Build history of the part. All positions in model axes, mm. Face numbers are marked on the shaded views. A direction names the side the tool comes from. Give positions to 0.01 mm unless a question says otherwise; leave off trailing zeros. Loops run counter-clockwise (first coordinate to the right, second up) from the corner with the lowest first, then second, coordinate; pieces in that order, holes last. Notation, with made-up numbers: M 33,78.25 L 62,78.25 A9 cw 62,93.25 Z; hole C 32,-17 d1. An arc over 180 degrees is marked long. Put each result on its own line as item: value.
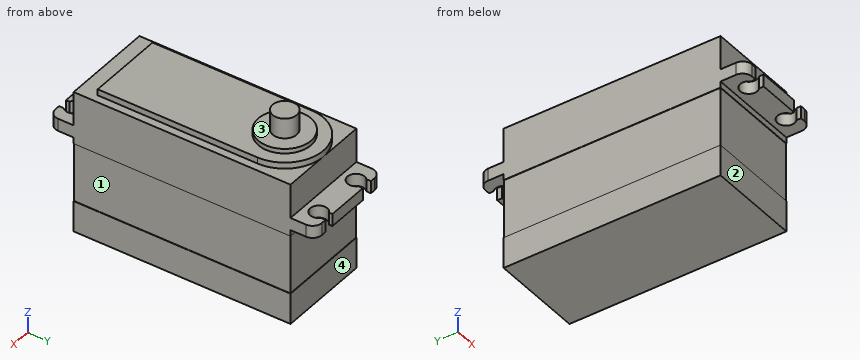
Autodesk Inventor part; units mm, degrees
ref_plane "Work Plane1" through (0, 0, 31) normal (0, 0, 1) x (1, 0, 0)
ref_plane "YZ Plane" through (0, 0, 0) normal (1, 0, 0) x (0, 1, 0)
ref_plane "XZ Plane" through (0, 0, 0) normal (0, 1, 0) x (-1, 0, 0)
sketch "Sketch1" plane through (0, 0, 0) normal (0, 0, 1) x (1, 0, 0)
  line L0 (0, 0) -> (-30, 0)
  line L1 (-30, 0) -> (-30, -70)
  line L2 (-30, -70) -> (0, -70)
  line L3 (0, -70) -> (0, 0)
  dimension "d0" = 30
  dimension "d1" = 70
extrude "Extrusion1" add sketch "Sketch1" along normal blind 10
sketch "Sketch2" plane through (0, 0, 10) normal (0, 0, 1) x (1, 0, 0)
  line L0 (-30, 0) -> (-30, -70)
  line L1 (-30, -70) -> (0, -70)
  line L2 (0, -70) -> (0, 0)
  line L3 (0, 0) -> (-30, 0)
  line L4 (0, 0) -> (-30, 0)
  line L5 (-30, -70) -> (0, -70)
  line L6 (-0.1, -70) -> (-0.1, -0.1)
  line L7 (-0.1, -0.1) -> (-30, -0.1)
  line L8 (-29.9, 0) -> (-29.9, -70)
  line L9 (-30, -69.9) -> (0, -69.9)
  point P0 (-29.9, -69.9)
  point P1 (-0.1, -69.9)
  point P2 (-29.9, -0.1)
  dimension "d29" = 0.1
  dimension "d30" = 0.1
  dimension "d31" = 0.1
extrude "Extrusion2" add sketch "Sketch2" along normal blind 19 contours L7 L6 L9 L8
sketch "Sketch3" plane through (0, 0, 29) normal (0, 0, 1) x (1, 0, 0)
  line L0 (-30, -70) -> (0, -70)
  line L1 (-30, 0) -> (-30, -70)
  line L2 (0, -70) -> (0, 0)
  line L3 (-30, -70) -> (0, -70)
  line L4 (0, 0) -> (-30, 0)
  line L5 (0, 0) -> (-30, 0)
  line L6 (0, -70) -> (0, 0)
  point P0 (-0.01, -70)
  point P1 (-0.01, 0)
extrude "Extrusion3" add sketch "Sketch3" along normal blind 19
sketch "Sketch4" plane through (0, 0, 48) normal (0, 0, 1) x (1, 0, 0)
  circle A0 centre (-15, -12.5) radius 8.5
  line L0 (0, 0) -> (-30, 0)
  dimension "d8" = 17
  dimension "d26" = 12.5
extrude "Extrusion4" add sketch "Sketch4" along normal blind 1.5
sketch "Sketch5" plane through (-15, -12.5, 49.5) normal (0, 0, 1) x (1, 0, 0)
  circle A0 centre (0, 0) radius 3.9
  point P0 (15, 12.5)
  dimension "d11" = 7.8
extrude "Extrusion5" add sketch "Sketch5" along normal blind 6.5
ref_plane "Work Plane1" through (0, 0, 31) normal (0, 0, 1) x (1, 0, 0)
sketch "Sketch6" plane through (0, 0, 31) normal (0, 0, 1) x (1, 0, 0)
  line L0 (-30, -70) -> (0, -70)
  line L1 (0, -70) -> (-30, -70)
  line L2 (-30, -70) -> (-30, -78)
  line L3 (0, -78) -> (0, -70)
  arc A0 (-4.6303, -76.5166) -> (-7.7916, -76.9278) centre (-6.5, -74.5) ccw
  arc A1 (-21.6303, -76.5166) -> (-25.3697, -76.5166) centre (-23.5, -74.5) ccw
  line L4 (-4.6303, -76.5166) -> (-4.6303, -78)
  line L5 (-7.7916, -76.9278) -> (-7.7916, -78)
  line L6 (-4.6303, -78) -> (0, -78)
  line L7 (-30, -78) -> (-25.3697, -78)
  line L8 (-21.6303, -78) -> (-7.7916, -78)
  line L9 (-21.6303, -76.5166) -> (-21.6303, -78)
  line L10 (-25.3697, -76.5166) -> (-25.3697, -78)
  line L11 (0, -70) -> (0, 0)
  line L12 (0, -35) -> (-30, -35) construction
  line L13 (-30, 0) -> (0, 0)
  line L14 (0, 0) -> (-30, 0)
  line L15 (-30, 0) -> (-30, 8)
  line L16 (0, 8) -> (0, 0)
  arc A2 (-7.7916, 6.9278) -> (-4.6303, 6.5166) centre (-6.5, 4.5) ccw
  arc A3 (-25.3697, 6.5166) -> (-21.6303, 6.5166) centre (-23.5, 4.5) ccw
  line L17 (-4.6303, 6.5166) -> (-4.6303, 8)
  line L18 (-7.7916, 6.9278) -> (-7.7916, 8)
  line L19 (-4.6303, 8) -> (0, 8)
  line L20 (-30, 8) -> (-25.3697, 8)
  line L21 (-21.6303, 8) -> (-7.7916, 8)
  line L22 (-21.6303, 6.5166) -> (-21.6303, 8)
  line L23 (-25.3697, 6.5166) -> (-25.3697, 8)
  point P0 (-0.01, -70)
  dimension "d15" = 30
  dimension "d16" = 8
  dimension "d17" = 5.5
  dimension "d18" = 5.5
  dimension "d21" = 6.5
  dimension "d22" = 6.5
extrude "Extrusion6" add sketch "Sketch6" along normal blind 4
fillet "Fillet1" radius 3 4 edges at (-30, 8, 33) (0, 8, 33) (-30, -78, 33) (0, -78, 33)
sketch "Sketch7" plane through (0, 0, 48) normal (0, 0, 1) x (1, 0, 0)
  point P0 (0, 0)
sketch "Sketch8" plane through (0, 0, 48) normal (0, 0, 1) x (1, 0, 0)
  circle A0 centre (-15, -12.5) radius 8.5
  circle A1 centre (-15, -12.5) radius 12.5
  line L0 (0, -70) -> (0, 0)
  line L1 (-2.5, -64) -> (-27.5, -64)
  line L2 (-30, 0) -> (-30, -70)
  line L3 (-2.5, -12.5) -> (-2.5, -64)
  line L4 (-27.5, -12.5) -> (-27.5, -64)
  line L5 (-30, -70) -> (0, -70)
  line L6 (0, 0) -> (-30, 0)
  point P0 (-15, 0)
extrude "Extrusion7" cut sketch "Sketch8" against normal blind 2 contours L6 L0 L5 L2
properties part number "serwo 30x70"
Q1. Slice it at A-A (y = -5). List the corners of the cut face in (x, z), and give its area (3 significant figures).
Here are the results:
outline: M -30,0 L 0,0 L 0,10 L -0.1,10 L -0.1,29 L 0,29 L 0,46 L -5,46 L -5,48 L -11,48 L -11,49.5 L -19,49.5 L -19,48 L -25,48 L -25,46 L -30,46 L -30,29 L -29.9,29 L -29.9,10 L -30,10 Z
area: 1,430 mm²
Q2. Drop flat-ended pins along their axis: pin 1 Ø6.5 at (x, y) = (-18, 2) entering from -Z; pin 2 Ø3.5 at (x, z) = (-22.5, 42.5) entering from -Y; pin 3 Ø2 at (x, z) = (-12.5, 17.5) entering from -Y; pin 4 Ø1.6 at (x, z) = (-20, 47) entering from -Y. Give the stop position or say it passes through.
Here are the results:
pin 1: z = 0
pin 2: y = -70
pin 3: y = -69.9
pin 4: y = -64
Q3. Probe line 1 (X direction, y = -74.5, z = 33.9); line 2 (Z direction, x = -14.5, y = -38); line 3 (Y direction, x = -16.75, z = 11). List the from-to ranges inside material, lowest first. Write a range as from..to.
Here are the results:
line 1: -30..-26.25, -20.75..-9.25, -3.75..0
line 2: 0..48
line 3: -69.9..-0.1
Q4. Tool access for the marked faces 1, 2, 3 and 4: list every direction of +Z, -Z, +X, -X, +Y, -Y with a clear straight run to the whole face (end or side of a thin tool).
Here are the results:
face 1: +X, +Y, -Y
face 2: -Z, +X, -X, -Y
face 3: +Z
face 4: -Z, +X, -X, +Y
Q5. Slice it at C-C (z = 5). List the corners of the cut face in (x, y), and give its area (3 significant figures).
Here are the results:
outline: M -30,-70 L 0,-70 L 0,0 L -30,0 Z
area: 2,100 mm²
Q6. Slice it at D-D (y = -38). List the corners of the cut face in (x, z), and give its area (3 significant figures).
Here are the results:
outline: M -30,0 L 0,0 L 0,10 L -0.1,10 L -0.1,29 L 0,29 L 0,46 L -2.5,46 L -2.5,48 L -27.5,48 L -27.5,46 L -30,46 L -30,29 L -29.9,29 L -29.9,10 L -30,10 Z
area: 1,430 mm²
